```python
from build123d import *

# Parameters (mm, degrees)
CHAMFER1_SIZE      = 1
SKETCH3_W          = 4
SKETCH3_H          = 4
CUT_EXTRUDE1_DEPTH = 10
CUT_EXTRUDE2_DEPTH = 10


with BuildPart() as part:
    # Sketch1 → Revolve1 (revolve)
    with BuildSketch(Plane.XY, mode=Mode.PRIVATE) as revolve1_sk:
        Polygon((-42.5, 0), (-42.5, 7.5), (-40.5, 7.5), (-40.5, 6), (-39, 6), (-39, 7.5), (39, 7.5), (39, 6), (40.5, 6), (40.5, 7.5), (42.5, 7.5), (42.5, 0), align=None)
    revolve(revolve1_sk.sketch.rotate(Axis((-47.151991765, 0, 0), (1, 0, 0)), 90), axis=Axis((-47.151991765, 0, 0), (1, 0, 0)))

    # Chamfer1
    chamfer1_edges = [part.edges().sort_by_distance(p)[0] for p in [
        (42.5, 0, -7.5),
        (-42.5, 0, -7.5),
    ]]
    chamfer(chamfer1_edges, length=CHAMFER1_SIZE)

    # Sketch3 → Cut-Extrude1 (cut)
    with BuildSketch(Plane(origin=(0, 0, 0), x_dir=(0, 0, -1), z_dir=(1, 0, 0))):
        with Locations((0, 7.5)):
            Rectangle(SKETCH3_W, SKETCH3_H)
    extrude(amount=-CUT_EXTRUDE1_DEPTH, mode=Mode.SUBTRACT)

    # Sketch4 → Cut-Extrude2 (cut)
    with BuildSketch(Plane(origin=(0, 5.5, 0), x_dir=(1, 0, 0), z_dir=(0, 1, 0))):
        with BuildLine():
            Line((27.5, -2), (-27.5, -2))
            ThreePointArc((-27.5, -2), (-29.5, 0), (-27.5, 2))
            Line((-27.5, 2), (27.5, 2))
            ThreePointArc((27.5, 2), (29.5, 0), (27.5, -2))
        make_face()
    extrude(amount=CUT_EXTRUDE2_DEPTH, mode=Mode.SUBTRACT)


solid = part.part
```
Build history of the part. All positions in model axes, mm. A direction names the side the tool comes from. Give positions to 0.01 mm unless a question says otherwise; leave off trailing zeros. Loops run counter-clockwise (first coordinate to the right, second up) from the corner with the lowest first, then second, coordinate; pieces in that order, holes last. Notation, with made-up numbers: (66.5, 33) -> (119.5, 33) arc R19 ccw to (119.5, 63) -> close; hole circle Ø7 at (16.5, 22.5). An arc over 180 degrees is marked (long way). One line per question, with ' | ' between items.
Q1. Tool access for faces 5 (the cylindrical face through (-39.74, -1.802, 5.723)), 6 (the flat face through (0, 6, -2)), 7 (the flat face through (-42.5, 0, 0)): list every direction of +Z, -Z, +X, -X, +Y, -Y with a clear straight run to the whole face (end or side of a thin tool).
Filled sheet:
face 5: none | face 6: +Y | face 7: +Z, -Z, -X, +Y, -Y
Q2. Cut at A-A, the plane z = 0. Write the cut outline in (x, y).
Filled sheet:
outline: (-42.5, -6.5) -> (-41.5, -7.5) -> (-40.5, -7.5) -> (-40.5, -6) -> (-39, -6) -> (-39, -7.5) -> (39, -7.5) -> (39, -6) -> (40.5, -6) -> (40.5, -7.5) -> (41.5, -7.5) -> (42.5, -6.5) -> (42.5, 6.5) -> (41.5, 7.5) -> (40.5, 7.5) -> (40.5, 6) -> (39, 6) -> (39, 7.5) -> (29.5, 7.5) -> (29.5, 5.5) -> (-29.5, 5.5) -> (-29.5, 7.5) -> (-39, 7.5) -> (-39, 6) -> (-40.5, 6) -> (-40.5, 7.5) -> (-41.5, 7.5) -> (-42.5, 6.5) -> close
Q3. Drop flat-ended pins along their axis: pin 1 (1.4 mm diameter, centred on x = -5, y = 6.5, fed in from -Z) (3 decimals); pin 2 (1.2 mm diameter, centred on x = -11.5, z = -0.5, fed in from +Y); pin 3 (1.5 mm diameter, centred on x = 11, z = 4.5, fed in from +Y). Give the stop position or say it passes through.
Filled sheet:
pin 1: stops at z = -4.755 | pin 2: stops at y = 5.5 | pin 3: stops at y = 6.5
Q4. Pull direction X, two halves, no side cores. Call faces 1 (the conical face through (-42, 0, -7)), 2 (the cylindrical face through (39.76, -1.802, 5.723)), 3 (the conical face through (42, 0, -7)), 4 (the flat face through (39, -6, 2)): pulls with the +X half, pulls with the -X half, needs draft (parallel to the pull), parting line crosses it, or undercut.
Filled sheet:
face 1: pulls with the -X half | face 2: undercut | face 3: pulls with the +X half | face 4: undercut
Q5. Drill centre lines: line 1 along X through (y, z) = (-5.5, -2.5); line 2 along X through (y, z) = (2.75, 6); line 3 along Z through (x, y) = (4, 0.25). Where is each one in solid material? Low to high. Write a range as [from, to].
Filled sheet:
line 1: x = [-42.5, -40.5], [-39, 39], [40.5, 42.5] | line 2: x = [-42.4, -40.5], [-39, 39], [40.5, 42.4] | line 3: z = [-7.5, 7.5]
Q6. Cut at B-B, the plane x = -31.5. Write the cut outline in (y, z), plus the area to 3 significant figures.
Filled sheet:
outline: circle Ø15 at (0, 0) | area: 177 mm²
Q7. Cut at C-C, the plane x = 25. Write the cut outline in (y, z).
Filled sheet:
outline: (5.5, -2) -> (5.5, 2) -> (7.23, 2) arc R7.5 ccw (long way) to (7.23, -2) -> close
